Geometry check sheet. Reference: the model listing, model coordinates, mm. A direction names the side the tool comes from. Coordinates: 2 decimals unless noted, no trailing zeros. Write each loop counter-clockwise with the first axis right and the second up, starting at its lowest first coordinate (ties: lowest second). Pieces come first, ordered by that corner, then holes. Notation, with made-up numbers: (29, -13) -> (73, -13) arc R18 ccw to (73, -2) -> close; hole circle Ø4 at (36.25, 43.25). An arc over 180 degrees is marked (long way). Put each result on its own line as item: value. Start each with the question number.
from build123d import *

# Parameters (mm, degrees)
F1_DEPTH = 200
F2_W     = 8.3923048454
F2_H     = 0.2
F3_DEPTH = 1
F2_W_2   = 0.9144346228
F2_H_2   = 1
F2_W_3   = 0.9401379739
F4_DEPTH = 2


with BuildPart() as f1:
    # F0 (on Front) → F1 (new body)
    with BuildSketch(Plane.XZ):
        with BuildLine():
            Line((-8, 0), (0, 0))
            Line((0, 0), (12, 0))
            Line((12, 0), (12, 1))
            ThreePointArc((12, 1), (6, 7), (0, 1))
            Line((0, 1), (0, 5))
            Line((0, 5), (-0.5, 5))
            Line((-0.5, 5), (-0.5, 1))
            Line((-0.5, 1), (-4.0740181695, 1))
            Line((-4.0740181695, 1), (-2.3419673619, 4))
            Line((-2.3419673619, 4), (-3.1502577388, 4))
            Line((-3.1502577388, 4), (-4.8823085464, 1))
            Line((-4.8823085464, 1), (-7.1917096231, 1))
            Line((-7.1917096231, 1), (-5.4596588156, 4))
            Line((-5.4596588156, 4), (-6.2679491924, 4))
            Line((-6.2679491924, 4), (-8, 1))
            Line((-8, 1), (-8, 0))
        make_face()
        with BuildLine():
            ThreePointArc((0.7, 1), (6, 6.3), (11.3, 1))
            Line((11.3, 1), (0.7, 1))
        make_face(mode=Mode.SUBTRACT)
    extrude(amount=F1_DEPTH)

    # F2 (on Front) → F3 (join)
    with BuildSketch(Plane.XZ):
        with BuildLine():
            ThreePointArc((0.9039230775, 1.2), (6, 6.1), (11.0960769225, 1.2))
            Line((11.0960769225, 1.2), (10.1961524227, 1.2))
            Line((10.1961524227, 1.2), (10.1961524227, 1))
            Line((10.1961524227, 1), (11.1105870456, 1))
            Line((11.1105870456, 1), (11.3, 1))
            ThreePointArc((11.3, 1), (6, 6.3), (0.7, 1))
            Line((0.7, 1), (0.8637096034, 1))
            Line((0.8637096034, 1), (1.8038475773, 1))
            Line((1.8038475773, 1), (1.8038475773, 1.2))
            Line((1.8038475773, 1.2), (0.9039230775, 1.2))
        make_face()
        with BuildLine():
            Line((10.1961524227, 1.2), (11.0960769225, 1.2))
            ThreePointArc((11.0960769225, 1.2), (6, 6.1), (0.9039230775, 1.2))
            Line((0.9039230775, 1.2), (1.8038475773, 1.2))
            Line((1.8038475773, 1.2), (10.1961524227, 1.2))
        make_face()
        with BuildLine():
            ThreePointArc((1.3384551917, 1.6), (6, 5.7), (10.6615448083, 1.6))
            Line((10.6615448083, 1.6), (1.3384551917, 1.6))
        make_face(mode=Mode.SUBTRACT)
        with Locations((6, 1.1)):
            Rectangle(F2_W, F2_H)
    extrude(amount=F3_DEPTH)

    # F2 (on Front) → F4 (join)
    with BuildSketch(Plane.XZ):
        with BuildLine():
            Line((10.1961524227, 1.2), (11.0960769225, 1.2))
            ThreePointArc((11.0960769225, 1.2), (6, 6.1), (0.9039230775, 1.2))
            Line((0.9039230775, 1.2), (1.8038475773, 1.2))
            Line((1.8038475773, 1.2), (10.1961524227, 1.2))
        make_face()
        with BuildLine():
            ThreePointArc((1.3384551917, 1.6), (6, 5.7), (10.6615448083, 1.6))
            Line((10.6615448083, 1.6), (1.3384551917, 1.6))
        make_face(mode=Mode.SUBTRACT)
        with Locations((10.6533697341, 0.5)):
            Rectangle(F2_W_2, F2_H_2)
        with Locations((1.3337785904, 0.5)):
            Rectangle(F2_W_3, F2_H_2)
        with BuildLine():
            ThreePointArc((0.9039230775, 1.2), (6, 6.1), (11.0960769225, 1.2))
            Line((11.0960769225, 1.2), (10.1961524227, 1.2))
            Line((10.1961524227, 1.2), (10.1961524227, 1))
            Line((10.1961524227, 1), (11.1105870456, 1))
            Line((11.1105870456, 1), (11.3, 1))
            ThreePointArc((11.3, 1), (6, 6.3), (0.7, 1))
            Line((0.7, 1), (0.8637096034, 1))
            Line((0.8637096034, 1), (1.8038475773, 1))
            Line((1.8038475773, 1), (1.8038475773, 1.2))
            Line((1.8038475773, 1.2), (0.9039230775, 1.2))
        make_face()
    extrude(amount=-F4_DEPTH)


solid = f1.part
Item 1: Go/stop test with flat-tipped pins: P1, Ø0.6, axis at x = -6, y = -137.5, coming from the +Z side; P2, Ø1.5, axis at x = -5, z = 5.5, coming from the -Y side; P3, Ø0.6, axis at x = 0, y = -81.5, coming from the +Z side; P4, Ø8, axis at x = -1.5, y = -122.5, coming from the +Z side. Record where each tip stops, or that it passes through.
Item 2: Section check B-B, the plane y = -132. Enter the section's corners in (x, z), and give its area (3 significant figures).
Item 3: Access from +Z, -Z, +X, -X, +Y, -Y to the whole of each face (thin tool, end or side, straight path). Record for faces 1 (the flat face through (2.7, -200, 0.7)), 2 (the flat face through (-0.5, -99, 3)).
Item 4: Mould release check, pull along Z, two halves, no side actions. Record for faces 3 (the flat face through (6, -99, 1)), 4 (the flat face through (6, -1, 1.3)), 5 (the cylindrical face through (6.1, 1, 6.3)), 6 (the flat face through (2, -100, 0)): released by +Z, released by -Z, zero draft, split by the parting line, or undercut.
Item 5: Section check A-A, the plane x = 6. Enter the section's corners in (y, z).
Item 6: Scan lines: line 1 along Z through (x, y) = (6.5, -188); line 2 along X through (y, z) = (-84.5, 4.5); line 3 along X through (y, z) = (-179, 4.75). Record each from-to range of solid material in increasing order. Write a range as [from, to].
From the geometry:
1. P1: z = 4
1. P2: through
1. P3: z = 5
1. P4: z = 5.87
2. outline: (-8, 0) -> (12, 0) -> (12, 1) arc R6 ccw to (0, 1) -> (0, 5) -> (-0.5, 5) -> (-0.5, 1) -> (-4.07, 1) -> (-2.34, 4) -> (-3.15, 4) -> (-4.88, 1) -> (-7.19, 1) -> (-5.46, 4) -> (-6.27, 4) -> (-8, 1) -> close; hole (0.7, 1) -> (11.3, 1) arc R5.3 ccw to start
2. area: 39.3 mm²
3. face 1: +Z, -Z, +X, -X, -Y
3. face 2: +Z, +Y, -Y
4. face 3: undercut
4. face 4: undercut
4. face 5: released by +Z
4. face 6: released by -Z
5. outline: (-200, 0) -> (0, 0) -> (0, 1.2) -> (2, 1.2) -> (2, 1.6) -> (-1, 1.6) -> (-1, 1) -> (-200, 1) -> close; (-200, 6.3) -> (-1, 6.3) -> (-1, 5.7) -> (2, 5.7) -> (2, 6.3) -> (0, 6.3) -> (0, 7) -> (-200, 7) -> close
6. line 1: [0, 1], [6.28, 6.98]
6. line 2: [-0.5, 0], [1.13, 2.02], [9.98, 10.87]
6. line 3: [-0.5, 0], [1.32, 2.25], [9.75, 10.68]
